from build123d import *

# Parameters (mm, degrees)
SKETCH1_R           = 122.75
SKETCH1_R_2         = 36
SKETCH1_W           = 20
SKETCH1_H           = 10
BOSS_EXTRUDE1_DEPTH = 10


with BuildPart() as part:
    # Sketch1 → Boss-Extrude1 (new body)
    with BuildSketch(Plane(origin=(0, 0, 0), x_dir=(1, 0, 0), z_dir=(0, 1, 0))):
        with Locations(Location((0, 0, 0), (0, 0, 270))):
            Circle(SKETCH1_R)
        with Locations(Location((0, 0, 0), (0, 0, 270))):
            Circle(SKETCH1_R_2, mode=Mode.SUBTRACT)
        with Locations((75, 0)):
            Rectangle(SKETCH1_W, SKETCH1_H, mode=Mode.SUBTRACT)
        with Locations((50, 0)):
            Rectangle(SKETCH1_W, SKETCH1_H, mode=Mode.SUBTRACT)
        with Locations((100, 0)):
            Rectangle(SKETCH1_W, SKETCH1_H, mode=Mode.SUBTRACT)
        Polygon((15.669872981, -37.141016151), (24.330127019, -32.141016151), (34.330127019, -49.461524227), (25.669872981, -54.461524227), align=None, mode=Mode.SUBTRACT)
        Polygon((28.169872981, -58.791651246), (36.830127019, -53.791651246), (46.830127019, -71.112159322), (38.169872981, -76.112159322), align=None, mode=Mode.SUBTRACT)
        Polygon((40.669872981, -80.442286341), (49.330127019, -75.442286341), (59.330127019, -92.762794416), (50.669872981, -97.762794416), align=None, mode=Mode.SUBTRACT)
        Polygon((-24.330127019, -32.141016151), (-15.669872981, -37.141016151), (-25.669872981, -54.461524227), (-34.330127019, -49.461524227), align=None, mode=Mode.SUBTRACT)
        Polygon((-36.830127019, -53.791651246), (-28.169872981, -58.791651246), (-38.169872981, -76.112159322), (-46.830127019, -71.112159322), align=None, mode=Mode.SUBTRACT)
        Polygon((-49.330127019, -75.442286341), (-40.669872981, -80.442286341), (-50.669872981, -97.762794416), (-59.330127019, -92.762794416), align=None, mode=Mode.SUBTRACT)
        with Locations((-50, 0)):
            Rectangle(SKETCH1_W, SKETCH1_H, mode=Mode.SUBTRACT)
        with Locations((-75, 0)):
            Rectangle(SKETCH1_W, SKETCH1_H, mode=Mode.SUBTRACT)
        with Locations((-100, 0)):
            Rectangle(SKETCH1_W, SKETCH1_H, mode=Mode.SUBTRACT)
        Polygon((-15.669872981, 37.141016151), (-24.330127019, 32.141016151), (-34.330127019, 49.461524227), (-25.669872981, 54.461524227), align=None, mode=Mode.SUBTRACT)
        Polygon((-28.169872981, 58.791651246), (-36.830127019, 53.791651246), (-46.830127019, 71.112159322), (-38.169872981, 76.112159322), align=None, mode=Mode.SUBTRACT)
        Polygon((-40.669872981, 80.442286341), (-49.330127019, 75.442286341), (-59.330127019, 92.762794416), (-50.669872981, 97.762794416), align=None, mode=Mode.SUBTRACT)
        Polygon((24.330127019, 32.141016151), (15.669872981, 37.141016151), (25.669872981, 54.461524227), (34.330127019, 49.461524227), align=None, mode=Mode.SUBTRACT)
        Polygon((36.830127019, 53.791651246), (28.169872981, 58.791651246), (38.169872981, 76.112159322), (46.830127019, 71.112159322), align=None, mode=Mode.SUBTRACT)
        Polygon((49.330127019, 75.442286341), (40.669872981, 80.442286341), (50.669872981, 97.762794416), (59.330127019, 92.762794416), align=None, mode=Mode.SUBTRACT)
    extrude(amount=BOSS_EXTRUDE1_DEPTH)


solid = part.part
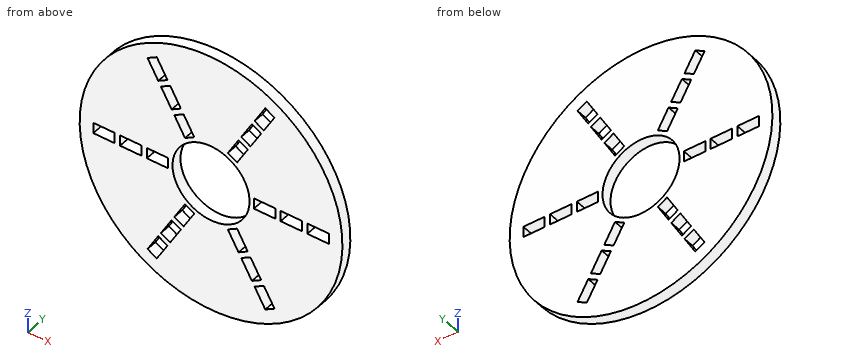
Read the model definition and answer for the solid it produces. Units are mm, in the model's axes. Give positions to 0.01 mm unless a question says otherwise; leave off trailing zeros. Write each loop counter-clockwise with the first axis right and the second up, starting at its lowest first coordinate (ties: lowest second). Pieces come first, ordered by that corner, then holes. Notation, with made-up numbers: (83, -9.5) - (97, -9.5) arc R32 ccw to (97, 29.5) - close; hole circle Ø9 at (-15.5, -2.5). An arc over 180 degrees is marked (long way). Use CSV: the item, a comma, the result in double quotes. Start each with the question number.
Item 1: Flat-ended cylindrical pins translate along their axes: P1, Ø3, axis at x = 72.5, y = 7.5, coming from the -Z side; P2, Ø3, axis at x = 78, y = 4.5, coming from the +Z side; P3, Ø1.5, axis at y = 4, z = -17.5, coming from the +X side. Find the tip coordinate at first contact, or state that the pin passes through.
Item 2: The part is cut by section A-A, the plane x = 0. Give the vertices of the cut face in (y, z), and give its area (4 significant figures).
Item 3: Consider line 1 (X direction, y = 8, z = 71.5); line 2 (Z direction, x = -18.5, y = 8); line 3 (X direction, y = 2.25, z = 83.5). Determine where each line is inside the solid, lowest interval first.
Item 4: The part is cut by section D-D, the plane x = 95. Give the vertices of the cut face in (y, z).
Item 5: The part is cut by section B-B, the plane z = 0. Count the separate pieces of the cut face and the enclosed holes in it, and give its area (3 significant figures).
Taken from the geometry:
1,P1,"z = -100.13"
1,P2,"z = 96"
1,P3,"x = 121.6"
2,outline,"(0, -122.75) - (10, -122.75) - (10, -36) - (0, -36) - close; (0, 36) - (10, 36) - (10, 122.75) - (0, 122.75) - close"
2,area,"1,735 mm2"
3,line 1,"-99.78 to -46.16, -35.51 to 35.51, 46.16 to 99.78"
3,line 2,"-121.35 to -42.04, -35.51 to -30.88, 30.88 to 35.51, 42.04 to 121.35"
3,line 3,"-89.97 to -53.98, -42.44 to 42.44, 53.98 to 89.97"
4,outline,"(0, -77.73) - (10, -77.73) - (10, -5) - (0, -5) - close; (0, 5) - (10, 5) - (10, 77.73) - (0, 77.73) - close"
5,separate pieces,"8"
5,enclosed holes,"0"
5,area,"535 mm2"
